```python
from build123d import *

# Parameters (mm, degrees)
F0_R     = 1.5875
F1_DEPTH = 2.54
F2_DEPTH = 2.54
F3_DEPTH = 1.651


with BuildPart() as f1:
    # F0 (on Top) → F1 (new body)
    with BuildSketch(Plane.XY):
        with BuildLine():
            ThreePointArc((-2.34618, 22.908559), (-2.870941, 22.729985), (-3.421944, 22.6695))
            Line((-3.421944, 22.6695), (-26.090599, 22.6695))
            ThreePointArc((-26.090599, 22.6695), (-26.641602, 22.729985), (-27.166363, 22.908559))
            Line((-27.166363, 22.908559), (-27.382744, 23.009724))
            ThreePointArc((-27.382744, 23.009724), (-29.832018, 25.031607), (-30.995815, 27.986693))
            Line((-30.995815, 27.986693), (-32.052543, 36.576))
            Line((-32.052543, 36.576), (-36.434043, 36.576))
            Line((-36.434043, 36.576), (-35.672043, 19.558))
            Line((-35.672043, 19.558), (-33.622761, 8.89))
            Line((-33.622761, 8.89), (-33.419602, 7.874))
            Line((-33.419602, 7.874), (3.915098, 7.874))
            Line((3.915098, 7.874), (4.110263, 8.89))
            Line((4.110263, 8.89), (6.1595, 19.558))
            Line((6.1595, 19.558), (6.9215, 36.576))
            Line((6.9215, 36.576), (2.54, 36.576))
            Line((2.54, 36.576), (1.483271, 27.986693))
            ThreePointArc((1.483271, 27.986693), (0.319475, 25.031607), (-2.129799, 23.009724))
            Line((-2.129799, 23.009724), (-2.34618, 22.908559))
        make_face()
        with Locations((-30.630143, 19.558)):
            Circle(F0_R, mode=Mode.SUBTRACT)
        with Locations((1.1176, 19.558)):
            Circle(F0_R, mode=Mode.SUBTRACT)
    extrude(amount=F1_DEPTH)

    # F0 (on Top) → F2 (join)
    with BuildSketch(Plane.XY):
        with BuildLine():
            Line((2.704744, 1.573093), (3.915098, 7.874))
            Line((3.915098, 7.874), (-33.419602, 7.874))
            Line((-33.419602, 7.874), (-32.152758, 1.5385))
            ThreePointArc((-32.152758, 1.5385), (-29.95333, -2.125914), (-25.9296, -3.566403))
            Line((-25.9296, -3.566403), (-24.686543, -3.567104))
            Line((-24.686543, -3.567104), (-24.686543, 2.233116))
            ThreePointArc((-24.686543, 2.233116), (-23.162543, 6.223), (-21.638543, 2.233116))
            Line((-21.638543, 2.233116), (-21.638543, -3.568821))
            Line((-21.638543, -3.568821), (-21.634144, -3.568824))
            Line((-21.634144, -3.568824), (-3.534824, -3.579023))
            ThreePointArc((-3.534824, -3.579023), (0.511873, -2.125521), (2.704744, 1.573093))
        make_face()
        Polygon((-1.27, 7.0104), (-1.27, -1.1176), (-14.478, -1.1176), (-17.018, 1.4224), (-17.018, 4.4704), (-14.478, 7.0104), align=None, mode=Mode.SUBTRACT)
    extrude(amount=F2_DEPTH)

    # F0 (on Top) → F3 (join)
    with BuildSketch(Plane.XY):
        with BuildLine():
            Line((2.704744, 1.573093), (3.915098, 7.874))
            Line((3.915098, 7.874), (-33.419602, 7.874))
            Line((-33.419602, 7.874), (-32.152758, 1.5385))
            ThreePointArc((-32.152758, 1.5385), (-29.95333, -2.125914), (-25.9296, -3.566403))
            Line((-25.9296, -3.566403), (-24.686543, -3.567104))
            Line((-24.686543, -3.567104), (-24.686543, 2.233116))
            ThreePointArc((-24.686543, 2.233116), (-23.162543, 6.223), (-21.638543, 2.233116))
            Line((-21.638543, 2.233116), (-21.638543, -3.568821))
            Line((-21.638543, -3.568821), (-21.634144, -3.568824))
            Line((-21.634144, -3.568824), (-3.534824, -3.579023))
            ThreePointArc((-3.534824, -3.579023), (0.511873, -2.125521), (2.704744, 1.573093))
        make_face()
        Polygon((-1.27, 7.0104), (-1.27, -1.1176), (-14.478, -1.1176), (-17.018, 1.4224), (-17.018, 4.4704), (-14.478, 7.0104), align=None, mode=Mode.SUBTRACT)
    extrude(amount=-F3_DEPTH)


solid = f1.part
```
The model under review builds one solid part; all positions refer to its coordinate system, in mm. A direction names the side the tool comes from. Give positions to 0.01 mm unless a question says otherwise; leave off trailing zeros. Write each loop counter-clockwise with the first axis right and the second up, starting at its lowest first coordinate (ties: lowest second). Pieces come first, ordered by that corner, then holes. Notation, with made-up numbers: M 31,63 L 53,63 A14 ccw 53,86 Z; hole C -4.5,-19.5 d1. An arc over 180 degrees is marked long. Write item = value, one per line. Start each with the question number.
Q1. Clearance check with flat-ended pins moving along their axes: pin 1 (2 mm diameter, centred on x = -18, y = 18.5, fed in from -Z); pin 2 (2 mm diameter, centred on y = -1.5, z = 0, fed in from -X); pin 3 (1.3 mm diameter, centred on x = -11, z = -0.5, fed in from -Y). State where each tip first meets the part, or that it passes through.
Q2. Machinability: for faces 1 (the face through (-21.639, -1, 0)), 2 (the face through (-26.634, 22.728, 1.252)), 3 (the face through (-15.77, 5.72, 0.47)), which of the approach directions +Z, -Z, +X, -X, +Y, -Y give a long, thin tool a straight path to every point of the face, cutting with its end or side? Answer none if there is none.
Q3. We need section D-D (y = 0). State the section outline as (x, z) points.
Q4. For line 1 (X direction, y = 1, z = 0.4); line 2 (Z direction, x = -22.5, y = 22); line 3 (Y direction, x = -20, z = 1.55), list the stretches that pass through material, from the lowest coordinate up.
Q5. Mouldability with a two-part tool opening along Y and no side actions: class faces 4 (the face through (-24.687, -1, 0)), 5 (the face through (-34.66, 14.3, 1.25)), 6 (the face through (-14, 7.874, -1)), 7 (the face through (-23.24, 6.22, 0.47)) as released by +Y, released by -Y, zero draft, split by the parting line, or undercut.
Q6. We need section B-B (x = -12). State the section outline as (y, z) points, plus the area to 3 significant figures.
Q7. We need section C-C (y = 30). State the section outline as (x, z) points, plus the area to 3 significant figures.
Result set:
q1.pin_1 = 0
q1.pin_2 = -31.36
q1.pin_3 = -3.58
q2.face_1 = +Z, -Z, -Y
q2.face_2 = +Z, -Z, +Y
q2.face_3 = +Z, -Z
q3.outline = M -31.63,-1.65 L -24.69,-1.65 L -24.69,2.54 L -31.63,2.54 Z; M -21.64,-1.65 L -15.6,-1.65 L -15.6,2.54 L -21.64,2.54 Z; M -1.27,-1.65 L 2.18,-1.65 L 2.18,2.54 L -1.27,2.54 Z
q4.line_1 = -32.02 to -24.69, -21.64 to -16.6, -1.27 to 2.57
q4.line_2 = 0 to 2.54
q4.line_3 = -3.57 to 22.67
q5.face_4 = zero draft
q5.face_5 = released by -Y
q5.face_6 = released by +Y
q5.face_7 = undercut
q6.outline = M -3.57,-1.65 L -1.12,-1.65 L -1.12,2.54 L -3.57,2.54 Z; M 7.01,-1.65 L 7.87,-1.65 L 7.87,0 L 22.67,0 L 22.67,2.54 L 7.01,2.54 Z
q6.area = 51.5 mm2
q7.outline = M -36.14,0 L -31.24,0 L -31.24,2.54 L -36.14,2.54 Z; M 1.73,0 L 6.63,0 L 6.63,2.54 L 1.73,2.54 Z
q7.area = 24.9 mm2
